The listing builds one solid part. Answer for the finished solid, in the listing's coordinates (mm). Give positions to 0.01 mm unless a question says otherwise; leave off trailing zeros. Loops run counter-clockwise (first coordinate to the right, second up) from the corner with the lowest first, then second, coordinate; pieces in that order, holes last. Notation, with made-up numbers: M 21,41 L 66,41 A16 ccw 66,51 Z; hole C -21,60.5 d3. An arc over 180 degrees is marked long. Return JSON: item names as keys, results as strings.
from build123d import *

# Parameters (mm, degrees)
EXTRUDE_1_DEPTH     = 10
SKETCH_3_R          = 2.5
CUT_EXTRUDE_1_DEPTH = 10
SKETCH_4_R          = 2.5
CUT_EXTRUDE_2_DEPTH = 10
SKETCH_5_R          = 2.5
CUT_EXTRUDE_3_DEPTH = 10


with BuildPart() as part:
    # 草图1 → 凸台-拉伸1 (new body)
    with BuildSketch(Plane.XY):
        with BuildLine():
            Line((-5, 0), (-5, 90))
            ThreePointArc((-5, 90), (0, 95), (5, 90))
            Line((5, 90), (5, 0))
            ThreePointArc((5, 0), (0, -5), (-5, 0))
        make_face()
    extrude(amount=EXTRUDE_1_DEPTH)

    # 草图3 → 切除-拉伸1 (cut)
    with BuildSketch(Plane(origin=(0, 0, 0), x_dir=(-1, 0, 0), z_dir=(0, 0, -1))):
        with Locations((0, 45)):
            Circle(SKETCH_3_R)
    extrude(amount=-CUT_EXTRUDE_1_DEPTH, mode=Mode.SUBTRACT)

    # 草图4 → 切除-拉伸2 (cut)
    with BuildSketch(Plane.XY.offset(10)):
        with Locations((0, 90)):
            Circle(SKETCH_4_R)
    extrude(amount=-CUT_EXTRUDE_2_DEPTH, mode=Mode.SUBTRACT)

    # 草图5 → 切除-拉伸3 (cut)
    with BuildSketch(Plane.XY.offset(10)):
        Circle(SKETCH_5_R)
    extrude(amount=-CUT_EXTRUDE_3_DEPTH, mode=Mode.SUBTRACT)


solid = part.part
(1) The part is cut by section A-A (y = 1.5). Determine the outline of the cut face in (x, z), and give its area (3 significant figures).
Values follow:
{"outline": "M -5,0 L -2,0 L -2,10 L -5,10 Z; M 2,0 L 5,0 L 5,10 L 2,10 Z", "area": "60.0 mm²"}
(2) The part is cut by section C-C (x = 0). Determine the outline of the cut face in (y, z).
Values follow:
{"outline": "M -5,0 L -2.5,0 L -2.5,10 L -5,10 Z; M 2.5,0 L 42.5,0 L 42.5,10 L 2.5,10 Z; M 47.5,0 L 87.5,0 L 87.5,10 L 47.5,10 Z; M 92.5,0 L 95,0 L 95,10 L 92.5,10 Z"}
(3) Straight lines are drawn through the part: line 1 along Y through (x, z) = (0, 7.75); line 2 along Y through (x, z) = (-0.75, 2); line 3 along X through (y, z) = (47, 6). For each, find the intervals that lie inside material, in ascending order.
Values follow:
{"line 1": "-5 to -2.5, 2.5 to 42.5, 47.5 to 87.5, 92.5 to 95", "line 2": "-4.94 to -2.38, 2.38 to 42.62, 47.38 to 87.62, 92.38 to 94.94", "line 3": "-5 to -1.5, 1.5 to 5"}
(4) The part is cut by section B-B (z = 6.25). Determine the outline of the cut face in (x, y).
Values follow:
{"outline": "M -5,0 A5 ccw 5,0 L 5,90 A5 ccw -5,90 Z; hole C 0,0 d5; hole C 0,45 d5; hole C 0,90 d5"}
(5) Given pin 1 (4.5 mm diameter, centred on x = 0, y = 90, fed in from +Z); pin 2 (1.5 mm diameter, centred on x = 2, z = 3.5, fed in from -Y), each flat-ended and moving along its own axis, determine where each tip first touches the part or whether it passes through.
Values follow:
{"pin 1": "through", "pin 2": "y = -4.84"}
(6) The part is cut by section D-D (y = 45). Determine the outline of the cut face in (x, z), and give its area (3 significant figures).
Values follow:
{"outline": "M -5,0 L -2.5,0 L -2.5,10 L -5,10 Z; M 2.5,0 L 5,0 L 5,10 L 2.5,10 Z", "area": "50.0 mm²"}
(7) Determine the mould class of faces 1 (the cylindrical face through (-0.54, -2.44, 5.07)), 2 (the cylindrical face through (0, -5, 5)), 3 (the flat face through (3, 46, 10)) for opening direction Y: released by +Y, released by -Y, zero draft, split by the parting line, or undercut.
Values follow:
{"face 1": "undercut", "face 2": "released by -Y", "face 3": "zero draft"}
